Build history of the part. All positions in model axes, mm. A direction names the side the tool comes from. Round coordinates to 2 decimals unless told otherwise and drop trailing zeros. Write each loop counter-clockwise with the first axis right and the second up, starting at its lowest first coordinate (ties: lowest second). Pieces come first, ordered by that corner, then holes. Notation, with made-up numbers: M 62,13.5 L 75,13.5 A29 cw 75,49.5 Z; hole C -26.5,80 d4. An arc over 180 degrees is marked long. Write item = value, one per line.
from build123d import *

# Parameters (mm, degrees)
F0_R     = 11.2
F0_R_2   = 13.2
F1_DEPTH = 7


with BuildPart() as f1:
    # F0 (on Top) → F1 (new body)
    with BuildSketch(Plane.XY):
        with BuildLine():
            ThreePointArc((26.475972, -1.993725), (13.469922, 5.91384), (8.528828, 20.310801))
            ThreePointArc((8.528828, 20.310801), (2.343248, 43.375827), (-11.511369, 23.925727))
            ThreePointArc((-11.511369, 23.925727), (-11.856497, 8.708375), (-21.854084, -2.769219))
            ThreePointArc((-21.854084, -2.769219), (-38.736192, -19.658602), (-14.964603, -21.932001))
            ThreePointArc((-14.964603, -21.932001), (-1.613425, -14.622215), (13.325256, -17.541582))
            ThreePointArc((13.325256, -17.541582), (36.392945, -23.717226), (26.475972, -1.993725))
        make_face()
        with Locations((-26.314595, -15.192739)):
            Circle(F0_R, mode=Mode.SUBTRACT)
        with Locations((26.314595, -15.192739)):
            Circle(F0_R, mode=Mode.SUBTRACT)
        Circle(F0_R_2, mode=Mode.SUBTRACT)
        with Locations((0, 30.385477)):
            Circle(F0_R, mode=Mode.SUBTRACT)
    extrude(amount=F1_DEPTH)


solid = f1.part
1. Band-saw the part on D-D (x = -30.5). List the corners of the cut face in (y, z).
Responses:
outline = M -27.71,0 L -25.58,0 L -25.58,7 L -27.71,7 Z; M -4.8,0 L -2.67,0 L -2.67,7 L -4.8,7 Z
2. Probe probe 1 along X at (y, z) = (-12, 4.25); probe 2 along Y at (x, z) = (-2, 1.5); probe 3 along Y at (x, z) = (0, 2). List the from-to ranges inside material, lowest first.
Responses:
probe_1 = -39.12 to -37.05, -15.58 to -5.5, 5.5 to 15.58, 37.05 to 39.12
probe_2 = -14.69 to -13.05, 13.05 to 19.37, 41.41 to 43.43
probe_3 = -14.43 to -13.2, 13.2 to 19.19, 41.59 to 43.59
3. Band-saw the part on B-B (x = 0). List the corners of the cut face in (y, z).
Responses:
outline = M -14.43,0 L -13.2,0 L -13.2,7 L -14.43,7 Z; M 13.2,0 L 19.19,0 L 19.19,7 L 13.2,7 Z; M 41.59,0 L 43.59,0 L 43.59,7 L 41.59,7 Z
4. Band-saw the part on C-C (y = -18.5). List the corners of the cut face in (x, z), plus the area to 3 significant figures.
Responses:
outline = M -39.09,0 L -37.02,0 L -37.02,7 L -39.09,7 Z; M -15.61,0 L -11.15,0 L -11.15,7 L -15.61,7 Z; M 13.54,0 L 15.61,0 L 15.61,7 L 13.54,7 Z; M 37.02,0 L 39.09,0 L 39.09,7 L 37.02,7 Z
area = 74.9 mm²
5. Tool access for faces 5 (the face through (2.753, 43.295, 3.451)), 6 (the face through (13.607, 5.745, 3.451)): list every direction of +Z, -Z, +X, -X, +Y, -Y with a clear straight run to the whole face (end or side of a thin tool).
Responses:
face_5 = +Z, -Z
face_6 = +Z, -Z, +X
6. Flat gauge pins, fed straight in: pin 1 (6 mm diameter, centred on x = 16.5, y = 32.5, fed in from -Z); pin 2 (4 mm diameter, centred on y = 0.5, z = 4, fed in from -X); pin 3 (1 mm diameter, centred on x = 6.5, z = 6, fed in from -Y); pin 4 (3 mm diameter, centred on y = -2, z = 5.5, fed in from -X). Where does each tip first touch, or does it go through?
Responses:
pin_1 = through
pin_2 = -19.83
pin_3 = -14.97
pin_4 = -32.44
7. Mould opens along Y. For faces 1 (the face through (-11.78, 8.91, 3.45)), 2 (the face through (-2.428, 19.452, 3.451)), 3 (the face through (36.12, -24.03, 3.45)), 4 (the face through (-1.828, -14.657, 3.451)) say: pulls with the +Y half, pulls with the -Y half, needs draft (parallel to the pull), parting line crosses it, or undercut.
Responses:
face_1 = undercut
face_2 = undercut
face_3 = parting line crosses it
face_4 = pulls with the -Y half
8. Band-saw the part on A-A (y = 26). List the corners of the cut face in (x, z), plus the area to 3 significant figures.
Responses:
outline = M -12.45,0 L -10.31,0 L -10.31,7 L -12.45,7 Z; M 10.31,0 L 12.45,0 L 12.45,7 L 10.31,7 Z
area = 30.0 mm²
